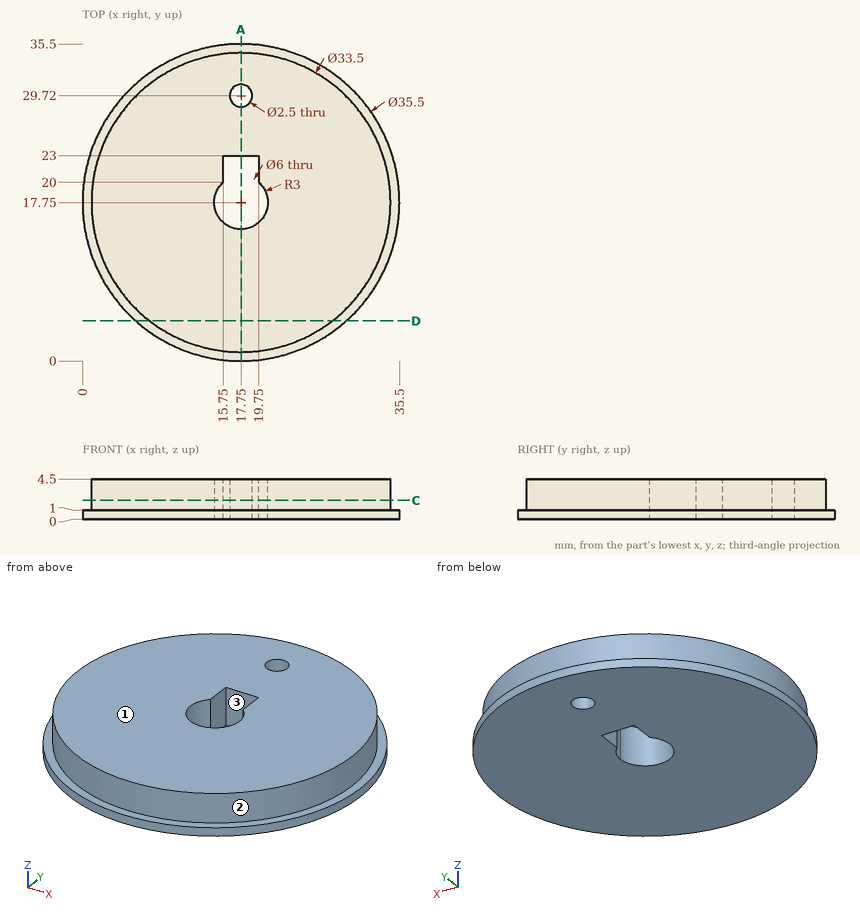
Design review of the part shown in the three views and the two pictorial views. Dimensions are in mm from the part's minimum x, y and z. Round coordinates to 2 decimals unless told otherwise and drop trailing zeros. Write each loop counter-clockwise with the first axis right and the second up, starting at its lowest first coordinate (ties: lowest second). Pieces come first, ordered by that corner, then holes. Notation, with made-up numbers: (4, 35) -> (53, 35) arc R14 ccw to (53, 42) -> close; hole circle Ø11 at (23.5, 89.25). An arc over 180 degrees is marked (long way). Use one line per item in the form item = value.
1) Take a section at C-C, the plane z = 2.1. Count the separate pieces of the cut face and the enclosed holes in it, and give its area (3 significant figures).
Found:
separate_pieces = 1
enclosed_holes = 2
area = 838 mm2
2) Clearance check with flat-ended pins moving along their axes: pin 1 (1.5 mm diameter, centred on x = 8, z = 2.5, fed in from +Y); pin 2 (1.2 mm diameter, centred on x = 18.5, z = 2.5, fed in from -Y); pin 3 (2.5 mm diameter, centred on y = 21.5, z = 2, fed in from +X) (1 decimal). State where each tip first meets the part, or that it passes through.
Found:
pin_1 = 31.88
pin_2 = 1
pin_3 = 35.2
3) Mouldability with a two-part tool opening along X and no side actions: class the marked faces 1, 2 and 3 as +X half, -X half, draft (parallel to the pull), parting line (faces both ways), or undercut.
Found:
face_1 = draft
face_2 = parting line
face_3 = undercut
4) To check wall thickness, follow L1, parallel to Y at x = 17.75, z = 2.1; L2, parallel to X at y = 30.5, z = 1.1 (1 decimal); L3, parallel to X at y = 11, z = 2.65. State the ranges of each line that lie inside material, in increasing order. Write a range as from..to.
Found:
L1 = 1..14.75, 23..28.47, 30.97..34.5
L2 = 6.9..16.8, 18.7..28.6
L3 = 2.42..33.08
5) Take a section at A-A, the plane x = 17.75. Write out the cut boundary in (y, z).
Found:
outline = (0, 0) -> (14.75, 0) -> (14.75, 4.5) -> (1, 4.5) -> (1, 1) -> (0, 1) -> close; (23, 0) -> (28.47, 0) -> (28.47, 4.5) -> (23, 4.5) -> close; (30.97, 0) -> (35.5, 0) -> (35.5, 1) -> (34.5, 1) -> (34.5, 4.5) -> (30.97, 4.5) -> close
6) Take a section at D-D, the plane y = 4.5. Write out the cut boundary in (x, z).
Found:
outline = (5.94, 0) -> (29.56, 0) -> (29.56, 1) -> (28, 1) -> (28, 4.5) -> (7.5, 4.5) -> (7.5, 1) -> (5.94, 1) -> close
